The listing builds one solid part. Answer for the finished solid, in the listing's coordinates (mm). A direction names the side the tool comes from. Round coordinates to 2 decimals unless told otherwise and drop trailing zeros. Order: outer loops, then holes, each group sorted by start corner. A loop starts at its lowest first (then second) coordinate and runs counter-clockwise, first axis right, second up. Notation, with made-up numbers: (-18, -28) -> (-1, -28) arc R14 ccw to (-1, -20) -> close; hole circle Ø4 at (-23.5, -15). An arc over 180 degrees is marked (long way). Answer in a Markdown table with one row per item. Add a question column.
```python
from build123d import *

# Parameters (mm, degrees)
F0_W      = 101.6
F0_H      = 76.2
F1_DEPTH  = 38.1
F2_T      = -3.81
F3_SIZE   = 10.16
F4_R      = 4.445
F4_R_2    = 1.27
F6_DEPTH  = 11.43
F5_R      = 4.445
F7_DEPTH  = 3.81
F8_W      = 12.7
F8_H      = 11.43
F9_DEPTH  = 3.81
F10_R     = 2.54
F11_R     = 5.08
F12_R     = 1.905
F13_DEPTH = 16.51


with BuildPart() as f1:
    # F0 (on Top) → F1 (new body)
    with BuildSketch(Plane.XY):
        with Locations((1.9488222897, 0.8362135466)):
            Rectangle(F0_W, F0_H)
    extrude(amount=F1_DEPTH)

    # F2
    f2_openings = [f1.faces().sort_by_distance(p)[0] for p in [
        (1.948822, 0.836214, 38.1),
    ]]
    offset(amount=F2_T, openings=f2_openings)

    # F3
    f3_edges = [f1.edges().sort_by_distance(p)[0] for p in [
        (-45.041178, 35.126214, 20.955),
        (48.938822, 35.126214, 20.955),
        (48.938822, -33.453786, 20.955),
        (-45.041178, -33.453786, 20.955),
    ]]
    chamfer(f3_edges, length=F3_SIZE)

    # F4 (on face) → F6 (join)
    with BuildSketch(Plane.XY.offset(3.81)):
        with Locations((-32.3411777103, -20.7537864534)):
            Circle(F4_R)
        with Locations((-32.3411777103, -20.7537864534)):
            Circle(F4_R_2, mode=Mode.SUBTRACT)
        with Locations((3.2188222897, 18.9762135466)):
            Circle(F4_R)
        with Locations((3.2188222897, 18.9762135466)):
            Circle(F4_R_2, mode=Mode.SUBTRACT)
    extrude(amount=F6_DEPTH)

    # F5 (on face) → F7 (cut, through all)
    with BuildSketch(Plane.YZ.offset(-45.0411777103)):
        with Locations((0.8362135466, 15.24)):
            Circle(F5_R)
    extrude(amount=-F7_DEPTH, mode=Mode.SUBTRACT)

    # F8 (on face) → F9 (cut, through all)
    with BuildSketch(Plane(origin=(0, -33.4537864534, 0), x_dir=(-1, 0, 0), z_dir=(0, 1, 0))):
        with Locations((14.6373170428, 12.7)):
            Rectangle(F8_W, F8_H)
    extrude(amount=-F9_DEPTH, mode=Mode.SUBTRACT)

    # F10
    f10_edges = [f1.edges().sort_by_distance(p)[0] for p in [
        (-8.287317, -35.358786, 6.985),
        (-20.987317, -35.358786, 6.985),
        (-20.987317, -35.358786, 18.415),
        (-8.287317, -35.358786, 18.415),
    ]]
    fillet(f10_edges, radius=F10_R)

    # F11
    f11_edges = [f1.edges().sort_by_distance(p)[0] for p in [
        (-48.851178, -37.263786, 19.05),
        (52.748822, -37.263786, 19.05),
        (52.748822, 38.936214, 19.05),
        (-48.851178, 38.936214, 19.05),
    ]]
    fillet(f11_edges, radius=F11_R)

    # F12 (on face) → F13 (cut)
    with BuildSketch(Plane.XY.offset(38.1)):
        with Locations((-43.7711777103, 33.8562135466)):
            Circle(F12_R)
        with Locations((-43.7711777103, -32.1837864534)):
            Circle(F12_R)
        with Locations((47.6688222897, 33.8562135466)):
            Circle(F12_R)
        with Locations((47.6688222897, -32.1837864534)):
            Circle(F12_R)
        with Locations((139.1088222897, 33.8562135466)):
            Circle(F12_R)
        with Locations((139.1088222897, -32.1837864534)):
            Circle(F12_R)
    extrude(amount=-F13_DEPTH, mode=Mode.SUBTRACT)


solid = f1.part
```
1. The part is cut by section A-A (x = -23.5). Give the vertices of the cut face in (y, z).
2. Each of these flat-tipped pins is pushed along its axis until it touches: pin 1 (10 mm diameter, centred on x = 2, y = 20, fed in from +Z); pin 2 (1.3 mm diameter, centred on x = -32.5, y = -21, fed in from +Z); pin 3 (1.1 mm diameter, centred on y = -35, z = 14, fed in from -X). Where does it stop, or does it pass through?
3. Straight lines are drawn through the part: line 1 along X through (y, z) = (-2, 20.5); line 2 along Y through (x, z) = (5, 16); line 3 along Y through (x, z) = (3, 11.5). For each, find the intervals that lie inside material, in ascending order.
4. For faces 1 (the flat face through (-8.287, -35, 13)), 2 (the flat face through (1, 38.936, 19)), 3 (the flat face through (2, 18, 15.24)), determine the directions among +Z, -Z, +X, -X, +Y, -Y from which every point of the face is accessible in a straight line to the end or side of a thin tool.
5. The part is cut by section B-B (y = -18). Give the vertices of the cut face in (x, z), then the cut area to 3 significant figures.
6. The part is cut by section C-C (y = -28). Give the vertices of the cut face in (x, z).
7. The mould has two halves that part along Z. Classify faces 4 (the flat face through (-15, -35, 18.415)), 5 (the flat face through (2, -36, 38.1)), 6 (the cylindrical face through (-47.4, 37.41, 19.32)): released by +Z, released by -Z, zero draft, split by the parting line, or undercut.
Report:
| question | item | result |
|---|---|---|
| 1 | outline | (-37.26, 0) -> (38.94, 0) -> (38.94, 38.1) -> (35.13, 38.1) -> (35.13, 3.81) -> (-33.45, 3.81) -> (-33.45, 38.1) -> (-37.26, 38.1) -> close |
| 2 | pin 1 | stops at z = 15.24 |
| 2 | pin 2 | stops at z = 3.81 |
| 2 | pin 3 | stops at x = -48.32 |
| 3 | line 1 | x = -48.85 to -45.04, 48.94 to 52.75 |
| 3 | line 2 | y = -37.26 to -33.45, 35.13 to 38.94 |
| 3 | line 3 | y = -37.26 to -33.45, 14.54 to 17.73, 20.23 to 23.42, 35.13 to 38.94 |
| 4 | face 1 | -Y |
| 4 | face 2 | +Z, -Z, +X, -X, +Y |
| 4 | face 3 | +Z |
| 5 | outline | (-48.85, 0) -> (52.75, 0) -> (52.75, 38.1) -> (48.94, 38.1) -> (48.94, 3.81) -> (-28.85, 3.81) -> (-28.85, 15.24) -> (-35.83, 15.24) -> (-35.83, 3.81) -> (-45.04, 3.81) -> (-45.04, 38.1) -> (-48.85, 38.1) -> close |
| 5 | area | 728 mm^2 |
| 6 | outline | (-48.85, 0) -> (52.75, 0) -> (52.75, 38.1) -> (44.23, 38.1) -> (44.23, 3.81) -> (-40.33, 3.81) -> (-40.33, 38.1) -> (-48.85, 38.1) -> close |
| 7 | face 4 | undercut |
| 7 | face 5 | released by +Z |
| 7 | face 6 | zero draft |
